The drawing under review shows one solid part. Ordinate dimensions are in mm from its lowest x, y, z. A direction names the side the tool comes from. Coordinates: 2 decimals unless noted, no trailing zeros. Write each loop counter-clockwise with the first axis right and the second up, starting at its lowest first coordinate (ties: lowest second). Pieces come first, ordered by that corner, then holes. Notation, with made-up numbers: (72, -36.5) -> (109, -36.5) arc R31 cw to (109, -0.5) -> close; hole circle Ø9 at (-19, -22.5). An arc over 180 degrees is marked (long way). One line per item, written item: value. Start each with the question number.
1) For pin 1 Ø3 at (y, z) = (5, 7) entering from +X; pin 2 Ø3.5 at (x, z) = (10, 10) entering from +Y; pin 3 Ø1.5 at (x, y) = (15, 2.5) entering from -Z, all flat-tipped, find the tip position at first contact; note any pin that passes through.
2) For probe 1 along Z at (x, y) = (10, 3.55); probe 2 along Z at (x, y) = (15, 4.25), list the stretches that pass through material, from the lowest coordinate up. Write a range as from..to.
3) Add section C-C (x = 10). State the section outline as (y, z) points, and give its area (3 significant figures).
4) Add section A-A (z = 10). State the section outline as (x, y) points.
5) Machinability: for the marked faces 4, 5 and 6, which of the approach directions +Z, -Z, +X, -X, +Y, -Y give a long, thin tool a straight path to every point of the face, cutting with its end or side? Answer none if there is none.
6) Add section D-D (z = 13.75). State the section outline as (x, y) points.
7) Add section B-B (y = 7). State the section outline as (x, z) points, and give its area (3 significant figures).
8) Mouldability with a two-part tool opening along Z and no side actions: class the marked faces 1, 2 and 3 as released by +Z, released by -Z, zero draft, split by the parting line, or undercut.
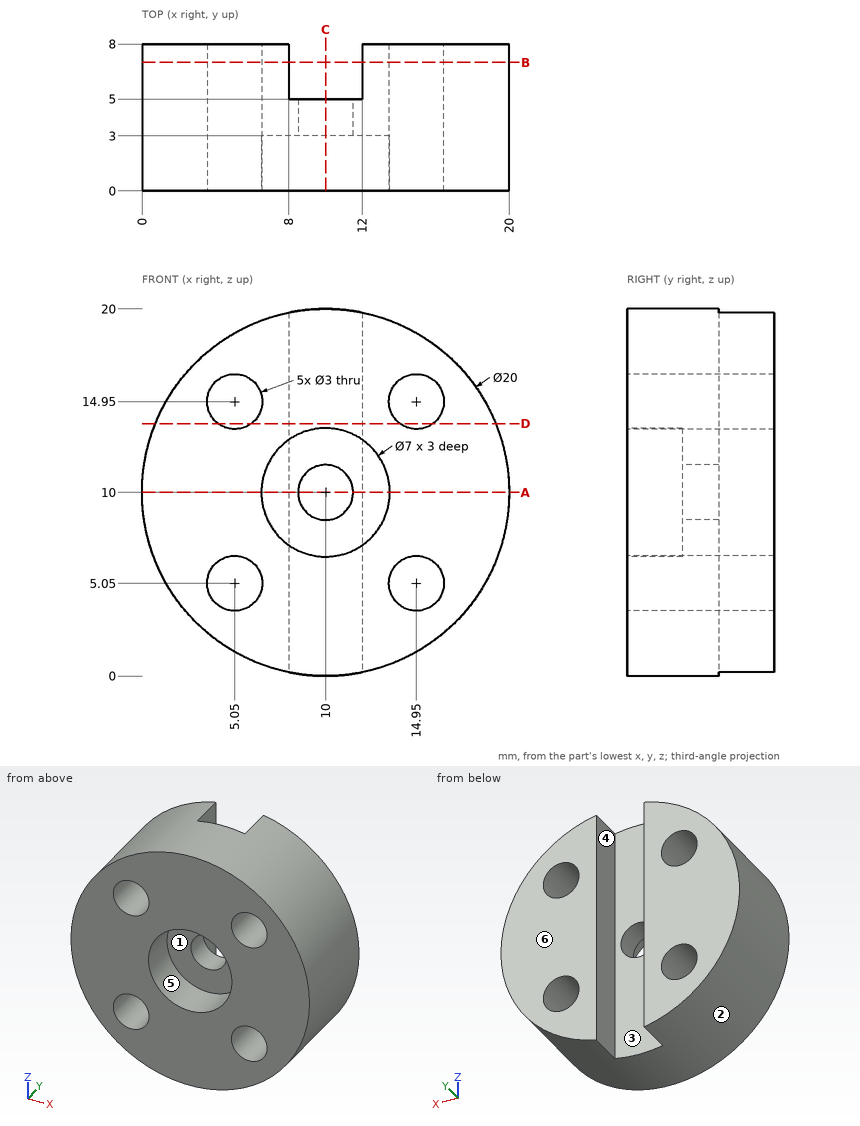
Numbers:
1. pin 1: x = 19.89
1. pin 2: y = 5
1. pin 3: z = 0.95
2. probe 1: 0..8.5, 11.5..20
2. probe 2: 1.34..3.55, 6.55..13.45, 16.45..18.66
3. outline: (0, 0) -> (5, 0) -> (5, 8.5) -> (3, 8.5) -> (3, 6.5) -> (0, 6.5) -> close; (0, 13.5) -> (3, 13.5) -> (3, 11.5) -> (5, 11.5) -> (5, 20) -> (0, 20) -> close
3. area: 73.0 mm²
4. outline: (0, 0) -> (6.5, 0) -> (6.5, 3) -> (8.5, 3) -> (8.5, 5) -> (8, 5) -> (8, 8) -> (0, 8) -> close; (11.5, 3) -> (13.5, 3) -> (13.5, 0) -> (20, 0) -> (20, 8) -> (12, 8) -> (12, 5) -> (11.5, 5) -> close
5. face 4: +Z, -Z, +Y
5. face 5: -Y
5. face 6: +Z, -Z, +X, -X, +Y
6. outline: (0.73, 0) -> (4.15, 0) -> (4.15, 8) -> (0.73, 8) -> close; (5.95, 0) -> (14.05, 0) -> (14.05, 8) -> (12, 8) -> (12, 5) -> (8, 5) -> (8, 8) -> (5.95, 8) -> close; (15.85, 0) -> (19.27, 0) -> (19.27, 8) -> (15.85, 8) -> close
7. outline: (8, 0.2) -> (8, 19.8) arc R10 ccw to start; (12, 0.2) arc R10 ccw to (12, 19.8) -> close; hole circle Ø3 at (5.05, 5.05); hole circle Ø3 at (5.05, 14.95); hole circle Ø3 at (14.95, 5.05); hole circle Ø3 at (14.95, 14.95)
7. area: 206 mm²
8. face 1: undercut
8. face 2: split by the parting line
8. face 3: zero draft
